Geometry check sheet. Reference: the model listing, model coordinates, mm. A direction names the side the tool comes from. Give positions to 0.01 mm unless a question says otherwise; leave off trailing zeros. Loops run counter-clockwise (first coordinate to the right, second up) from the corner with the lowest first, then second, coordinate; pieces in that order, holes last. Notation, with made-up numbers: (28.5, 84.25) -> (76.5, 84.25) arc R20 cw to (76.5, 119.25) -> close; hole circle Ø3 at (46.25, 32). An arc over 180 degrees is marked (long way). One line per item, written item: value. Start each with the question number.
(1) Sectioned sample at B-B, the plane x = 0. Record the cut outline in (y, z) (1 decimal).
(2) Sectioned sample at A-A, the plane y = 0. Record the cut outline in (x, z) (3 decimals), then the cut area to 3 significant figures.
(3) Scan lines: line 1 along X through (y, z) = (8.5, -31) (1 decimal); line 2 along Y through (x, z) = (3.5, 27); line 3 along Z through (x, y) = (19, 5) (3 decimals). Record each from-to range of solid material in increasing order. Write a range as from..to.
(4) Tool access check on faces 1 (the face through (17.95, 0, 39)), 2 (the face through (-11.4, 17.1, 0)), 3 (the face through (10, 0, 76.2)), 4 (the face through (4, -17.318, 39)), 5 (the face through (-7.96, 9.5, 13.59)). Record the directions out of +Z, -Z, +X, -X, +Y, -Y that give a thin tool (end or side, any length) a straight path to the whole face; none if there is none.
(5) Gauge pin test, flat ends, axial feed: pin 1 Ø12.5 at (x, z) = (-0.5, 28) entering from -Y; pin 2 Ø10 at (x, z) = (7.5, 37.5) entering from +Y; pin 3 Ø2 at (x, y) = (19, 15.5) entering from +Z (3 decimals). Record the tip position at first contact, or that the pin passes through.
(6) Draft check along Y on faces 6 (the face through (13, 0, -50.8)), 7 (the face through (-9.633, -12, 14)), 8 (the face through (2, -11.112, 14)), 9 (the face through (4, 17.634, 39)). Enter one of: pulls with the +Y half, pulls with the -Y half, needs draft (parallel to the pull), parting line crosses it, or undercut.
from build123d import *

# Parameters (mm, degrees)
F0_R          = 20.32
F0_R_2        = 17.145
F2_DEPTH      = 50.8
F1_R          = 25.4
F1_R_2        = 17.145
F3_DEPTH      = 3.175
F4_W          = 27.5823939592
F4_H          = 34.9517390132
F5_DEPTH      = 76.2
F5_DEPTH_BACK = 50.8
F6_R          = 34.0814213396
F6_R_2        = 20.32
F7_DEPTH      = 76.2
F8_W          = 9.0154311216
F8_H          = 15.875
F9_DEPTH      = 76.2
F9_DEPTH_BACK = 76.2


with BuildPart() as f2:
    # F0 (on Top) → F2 (new body)
    with BuildSketch(Plane.XY):
        Circle(F0_R)
        Circle(F0_R_2, mode=Mode.SUBTRACT)
    extrude(amount=-F2_DEPTH)

    # F1 (on Top) → F3 (join)
    with BuildSketch(Plane.XY):
        Circle(F1_R)
        Circle(F1_R_2, mode=Mode.SUBTRACT)
    extrude(amount=F3_DEPTH)

    # F4 (on Top) → F5 (join, two sides)
    with BuildSketch(Plane.XY) as f5_sk:
        with Locations((4.1584149003, 0.1579150558)):
            Rectangle(F4_W, F4_H)
        Polygon((9.525, 11.1125), (9.525, -11.1125), (-6.35, -11.1125), (-9.525, -11.1125), (-9.525, -7.9375), (-9.525, 7.9375), (-9.525, 11.1125), (-6.35, 11.1125), align=None, mode=Mode.SUBTRACT)
        Polygon((-9.525, -11.1125), (-6.35, -11.1125), (-9.525, -7.9375), align=None)
        Polygon((-9.525, 7.9375), (-6.35, 11.1125), (-9.525, 11.1125), align=None)
    extrude(amount=F5_DEPTH)
    extrude(f5_sk.sketch, amount=-F5_DEPTH_BACK)

    # F6 (on Top) → F7 (cut)
    with BuildSketch(Plane.XY):
        Circle(F6_R)
        Circle(F6_R_2, mode=Mode.SUBTRACT)
    extrude(amount=-F7_DEPTH, mode=Mode.SUBTRACT)

    # F8 (on Top) → F9 (cut, two sides)
    with BuildSketch(Plane.XY) as f9_sk:
        with Locations((-7.6543868054, -0.1444227528)):
            Rectangle(F8_W, F8_H)
    extrude(amount=-F9_DEPTH, mode=Mode.SUBTRACT)
    extrude(f9_sk.sketch, amount=F9_DEPTH_BACK, mode=Mode.SUBTRACT)


solid = f2.part
Calculated:
1. outline: (-25.4, 0) -> (-20.3, 0) -> (-20.3, -50.8) -> (-11.1, -50.8) -> (-11.1, 76.2) -> (-17.3, 76.2) -> (-17.3, 3.2) -> (-25.4, 3.2) -> close; (11.1, -50.8) -> (20.3, -50.8) -> (20.3, 0) -> (25.4, 0) -> (25.4, 3.2) -> (17.6, 3.2) -> (17.6, 76.2) -> (11.1, 76.2) -> close
2. outline: (-25.4, 0) -> (-20.32, 0) -> (-20.32, -50.8) -> (-17.145, -50.8) -> (-17.145, 3.175) -> (-25.4, 3.175) -> close; (9.525, -50.8) -> (20.32, -50.8) -> (20.32, 0) -> (25.4, 0) -> (25.4, 3.175) -> (17.95, 3.175) -> (17.95, 76.2) -> (9.525, 76.2) -> close
2. area: 1,400 mm2
3. line 1: x = -18.5..-14.9, -9.6..-9, 9.5..18.5
3. line 2: y = -17.32..-11.11, 11.11..17.63
3. line 3: z = -50.8..3.175
4. face 1: +Z, +X, +Y, -Y
4. face 2: -Z
4. face 3: +Z, +X, -X, +Y, -Y
4. face 4: +Z, +X, -X, -Y
4. face 5: +Z, -Z
5. pin 1: stops at y = -17.32
5. pin 2: stops at y = 17.63
5. pin 3: stops at z = 3.175
6. face 6: needs draft
6. face 7: undercut
6. face 8: undercut
6. face 9: pulls with the +Y half
